```python
from build123d import *

# Parameters (mm, degrees)
F0_W          = 30
F0_H          = 42
F1_DEPTH      = 5
F2_T1_DEPTH   = 186.6590212458
F3_W          = 30
F3_H          = 2
F4_DEPTH      = 10
F5_W          = 35
F5_H          = 30
F6_DEPTH      = 5
F7_W          = 7
F7_H          = 30
F8_DEPTH      = 15
F9_R          = 2
F10_DEPTH     = 10
F11_R         = 4
F12_W         = 15
F12_H         = 14
F13_DEPTH     = 5
F14_W         = 15
F14_H         = 15
F15_DEPTH     = 5
F16_T4_DEPTH  = 35.8601958556
F16_T9_DEPTH  = 35.8601958556
F17_R         = 5
F18_T1_DEPTH  = 20
F18_T6_DEPTH  = 9.5699020722
F18_T11_DEPTH = 31.2132034356
F18_T16_DEPTH = 31.2132034356
F18_T21_DEPTH = 14
F18_T24_ANGLE = 90
F18_T26_ANGLE = 90
F18_T30_DEPTH = 13
F18_T36_DEPTH = 14
F18_T40_DEPTH = 31.2132034356
F18_T47_DEPTH = 13
F18_T51_DEPTH = 31.2132034356


# Not quite as in the source:
# - a fillet or chamfer that OpenCascade refuses, or shapes differently, is made with other operations: its cross-section is extruded or revolved along the edge and cut away or added


with BuildPart() as f1:
    # F0 (on Top) → F1 (new body)
    with BuildSketch(Plane.XY):
        with Locations((15, 21)):
            Rectangle(F0_W, F0_H)
    extrude(amount=F1_DEPTH)

    # F2: fillet of radius 37 on 1 edges, made by hand

    # F2_s2 → F2_t1 (cut)
    with BuildSketch(Plane.XY.offset(-90.8295106229)):
        with BuildLine():
            ThreePointArc((30, 5.6681957508), (21.5306852354, 29.2266337296), (0, 42))
            Line((0, 42), (30, 42))
            Line((30, 42), (30, 5.6681957508))
        make_face()
    extrude(amount=F2_T1_DEPTH, mode=Mode.SUBTRACT)

    # F3 (on face) → F4 (join)
    with BuildSketch(Plane.XY.offset(5)):
        with Locations((15, 1)):
            Rectangle(F3_W, F3_H)
    extrude(amount=F4_DEPTH)

    # F5 (on face) → F6 (join)
    with BuildSketch(Plane(origin=(0, 0, 0), x_dir=(0, -1, 0), z_dir=(-1, 0, 0))):
        with Locations((-25.5, 15)):
            Rectangle(F5_W, F5_H)
    extrude(amount=F6_DEPTH)

    # F7 (on face) → F8 (join)
    with BuildSketch(Plane(origin=(-5, 0, 0), x_dir=(0, -1, 0), z_dir=(-1, 0, 0))):
        with Locations((-11.5, 15)):
            Rectangle(F7_W, F7_H)
    extrude(amount=F8_DEPTH)

    # F9 (on face) → F10 (cut)
    with BuildSketch(Plane(origin=(0, 15, 0), x_dir=(-1, 0, 0), z_dir=(0, 1, 0))):
        with Locations((10, 15)):
            Circle(F9_R)
    extrude(amount=-F10_DEPTH, mode=Mode.SUBTRACT)

    # F11
    f11_edges = [f1.edges().sort_by_distance(p)[0] for p in [
        (21.530685, 29.226634, 0),
        (15, 0, 0),
    ]]
    fillet(f11_edges, radius=F11_R)

    # F12 (on face) → F13 (join)
    with BuildSketch(Plane(origin=(0, 0, 0), x_dir=(1, 0, 0), z_dir=(0, 0, -1))):
        with Locations((-12.5, -22)):
            Rectangle(F12_W, F12_H)
    extrude(amount=-F13_DEPTH)

    # F14 (on face) → F15 (join)
    with BuildSketch(Plane.XY.offset(30)):
        with Locations((-12.5, 22.5)):
            Rectangle(F14_W, F14_H)
    extrude(amount=-F15_DEPTH)

    # F16: chamfer of 15 on 2 edges, made by hand


with BuildPart() as f16_tool2:
    # F16_s3 → F16_t4 (new body)
    with BuildSketch(Plane.XY.offset(45.4300979278)):
        with BuildLine():
            Line((-20.4242640687, 14.5757359313), (-4.5757359313, 30.4242640687))
            Line((-4.5757359313, 30.4242640687), (-4.5757359313, 30.7242640687))
            ThreePointArc((-4.5757359313, 30.7242640687), (-12.2878679656, 30.3), (-20, 30.3))
            Line((-20, 30.3), (-20.3, 30))
            ThreePointArc((-20.3, 30), (-20.3, 22.2878679656), (-20.7242640687, 14.5757359313))
            Line((-20.7242640687, 14.5757359313), (-20.4242640687, 14.5757359313))
        make_face()
    extrude(amount=-F16_T4_DEPTH)

    split(bisect_by=Plane.YZ.offset(-5), keep=Keep.BOTTOM)


with BuildPart() as f1_1:
    add(f1.part)

    # F16_t1: cut F16_tool2
    add(f16_tool2.part, mode=Mode.SUBTRACT)


with BuildPart() as f16_tool7:
    # F16_s8 → F16_t9 (new body)
    with BuildSketch(Plane.XY.offset(-15.4300979278)):
        with BuildLine():
            Line((-4.5757359313, 29.4242640687), (-20.4242640687, 13.5757359313))
            Line((-20.4242640687, 13.5757359313), (-20.7242640687, 13.5757359313))
            ThreePointArc((-20.7242640687, 13.5757359313), (-20.3, 21.2878679656), (-20.3, 29))
            Line((-20.3, 29), (-20, 29.3))
            ThreePointArc((-20, 29.3), (-12.2878679656, 29.3), (-4.5757359313, 29.7242640687))
            Line((-4.5757359313, 29.7242640687), (-4.5757359313, 29.4242640687))
        make_face()
    extrude(amount=F16_T9_DEPTH)

    split(bisect_by=Plane.YZ.offset(-5), keep=Keep.BOTTOM)


with BuildPart() as f1_2:
    add(f1_1.part)

    # F16_t6: cut F16_tool7
    add(f16_tool7.part, mode=Mode.SUBTRACT)

    # F17
    f17_edges = [f1_2.edges().sort_by_distance(p)[0] for p in [
        (-2.5, 43, 0),
        (-2.5, 43, 30),
    ]]
    fillet(f17_edges, radius=F17_R)

    # F18: fillet of radius 2 on 9 edges, made by hand

    # F18_s2 → F18_t1 (cut)
    with BuildSketch(Plane.XY.offset(5)):
        with BuildLine():
            ThreePointArc((-3, 43), (-4.4142135624, 42.4142135624), (-5, 41))
            Line((-5, 41), (-5, 43))
            Line((-5, 43), (-3, 43))
        make_face()
    extrude(amount=F18_T1_DEPTH, mode=Mode.SUBTRACT)


with BuildPart() as f18_tool4:
    # F18_s5 → F18_t6 (new body)
    with BuildSketch(Plane.XY.offset(25)):
        with BuildLine():
            ThreePointArc((-20, 13), (-19.4142135624, 14.4142135624), (-18, 15))
            Line((-18, 15), (-20, 15))
            Line((-20, 15), (-20, 13))
        make_face()
    extrude(amount=-F18_T6_DEPTH)

    split(bisect_by=Plane(origin=(-17, 17, 0), x_dir=(0, 0, 1), z_dir=(-0.7071067812, 0.7071067812, 0)), keep=Keep.TOP)


with BuildPart() as f1_3:
    add(f1_2.part)

    # F18_t3: cut F18_tool4
    add(f18_tool4.part, mode=Mode.SUBTRACT)


with BuildPart() as f18_tool9:
    # F18_s10 → F18_t11 (new body)
    with BuildSketch(Plane(origin=(-6.5355339059, -6.5355339059, 0), x_dir=(0, 0, 1), z_dir=(0.7071067812, 0.7071067812, 0))):
        with BuildLine():
            ThreePointArc((0, -22.0416305603), (0.5857864376, -23.4558441227), (2, -24.0416305603))
            Line((2, -24.0416305603), (0, -24.0416305603))
            Line((0, -24.0416305603), (0, -22.0416305603))
        make_face()
    extrude(amount=F18_T11_DEPTH)

    split(bisect_by=Plane.YZ.offset(-5), keep=Keep.BOTTOM)


with BuildPart() as f1_4:
    add(f1_3.part)

    # F18_t8: cut F18_tool9
    add(f18_tool9.part, mode=Mode.SUBTRACT)


with BuildPart() as f18_tool14:
    # F18_s15 → F18_t16 (new body)
    with BuildSketch(Plane(origin=(16.0355339059, 16.0355339059, 0), x_dir=(0, 0, 1), z_dir=(-0.7071067812, -0.7071067812, 0))):
        with BuildLine():
            ThreePointArc((30, 22.7487373415), (29.4142135624, 24.1629509039), (28, 24.7487373415))
            Line((28, 24.7487373415), (30, 24.7487373415))
            Line((30, 24.7487373415), (30, 22.7487373415))
        make_face()
    extrude(amount=F18_T16_DEPTH)

    split(bisect_by=Plane.YZ.offset(-5), keep=Keep.BOTTOM)


with BuildPart() as f1_5:
    add(f1_4.part)

    # F18_t13: cut F18_tool14
    add(f18_tool14.part, mode=Mode.SUBTRACT)


with BuildPart() as f18_tool19:
    # F18_s20 → F18_t21 (new body)
    with BuildSketch(Plane.XZ.offset(-24)):
        with BuildLine():
            ThreePointArc((-3, 0), (-4.4142135624, 0.5857864376), (-5, 2))
            Line((-5, 2), (-5, 0))
            Line((-5, 0), (-3, 0))
        make_face()
    extrude(amount=-F18_T21_DEPTH)

    split(bisect_by=Plane(origin=(-17, 17, 0), x_dir=(0, 0, 1), z_dir=(-0.7071067812, 0.7071067812, 0)), keep=Keep.TOP)


with BuildPart() as f1_6:
    add(f1_5.part)

    # F18_t18: cut F18_tool19
    add(f18_tool19.part, mode=Mode.SUBTRACT)

    # F18_s23 → F18_t24 (revolve, cut)
    with BuildSketch(Plane.XY.offset(5)):
        with BuildLine():
            ThreePointArc((-3, 43), (-4.4142135624, 42.4142135624), (-5, 41))
            Line((-5, 41), (-5, 43))
            Line((-5, 43), (-3, 43))
        make_face()
    revolve(axis=Axis((-5, 38, 5), (-1, 0, 0)), revolution_arc=F18_T24_ANGLE, mode=Mode.SUBTRACT)

    # F18_s25 → F18_t26 (revolve, cut)
    with BuildSketch(Plane.XY.offset(25)):
        with BuildLine():
            ThreePointArc((-3, 43), (-4.4142135624, 42.4142135624), (-5, 41))
            Line((-5, 41), (-5, 43))
            Line((-5, 43), (-3, 43))
        make_face()
    revolve(axis=Axis((-5, 38, 25), (1, 0, 0)), revolution_arc=F18_T26_ANGLE, mode=Mode.SUBTRACT)


with BuildPart() as f18_tool28:
    # F18_s29 → F18_t30 (new body)
    with BuildSketch(Plane.XZ.offset(-25)):
        with BuildLine():
            ThreePointArc((-3, 30), (-4.4142135624, 29.4142135624), (-5, 28))
            Line((-5, 28), (-5, 30))
            Line((-5, 30), (-3, 30))
        make_face()
    extrude(amount=-F18_T30_DEPTH)

    split(bisect_by=Plane(origin=(-17.5, 17.5, 0), x_dir=(0, 0, 1), z_dir=(-0.7071067812, 0.7071067812, 0)), keep=Keep.TOP)


with BuildPart() as f1_7:
    add(f1_6.part)

    # F18_t27: cut F18_tool28
    add(f18_tool28.part, mode=Mode.SUBTRACT)


with BuildPart() as f18_tool34:
    # F18_s35 → F18_t36 (new body)
    with BuildSketch(Plane.XZ.offset(-24)):
        with BuildLine():
            ThreePointArc((-3, 0), (-4.4142135624, 0.5857864376), (-5, 2))
            Line((-5, 2), (-5, 0))
            Line((-5, 0), (-3, 0))
        make_face()
    extrude(amount=-F18_T36_DEPTH)

    split(bisect_by=Plane(origin=(-17, 17, 0), x_dir=(0, 0, 1), z_dir=(0.7071067812, -0.7071067812, 0)), keep=Keep.TOP)


with BuildPart() as f18_tool38:
    # F18_s39 → F18_t40 (new body)
    with BuildSketch(Plane(origin=(-6.5355339059, -6.5355339059, 0), x_dir=(0, 0, 1), z_dir=(0.7071067812, 0.7071067812, 0))):
        with BuildLine():
            ThreePointArc((0, -22.0416305603), (0.5857864376, -23.4558441227), (2, -24.0416305603))
            Line((2, -24.0416305603), (0, -24.0416305603))
            Line((0, -24.0416305603), (0, -22.0416305603))
        make_face()
    extrude(amount=F18_T40_DEPTH)

    split(bisect_by=Plane.YZ.offset(-5), keep=Keep.TOP)


with BuildPart() as f18_tool34_1:
    add(f18_tool34.part)

    # F18_t42: intersect F18_tool38
    add(f18_tool38.part, mode=Mode.INTERSECT)


with BuildPart() as f1_8:
    add(f1_7.part)

    # F18_t32: cut F18_tool34
    add(f18_tool34_1.part, mode=Mode.SUBTRACT)


with BuildPart() as f18_tool45:
    # F18_s46 → F18_t47 (new body)
    with BuildSketch(Plane.XZ.offset(-25)):
        with BuildLine():
            ThreePointArc((-3, 30), (-4.4142135624, 29.4142135624), (-5, 28))
            Line((-5, 28), (-5, 30))
            Line((-5, 30), (-3, 30))
        make_face()
    extrude(amount=-F18_T47_DEPTH)

    split(bisect_by=Plane(origin=(-17.5, 17.5, 0), x_dir=(0, 0, 1), z_dir=(0.7071067812, -0.7071067812, 0)), keep=Keep.TOP)


with BuildPart() as f18_tool49:
    # F18_s50 → F18_t51 (new body)
    with BuildSketch(Plane(origin=(16.0355339059, 16.0355339059, 0), x_dir=(0, 0, 1), z_dir=(-0.7071067812, -0.7071067812, 0))):
        with BuildLine():
            ThreePointArc((30, 22.7487373415), (29.4142135624, 24.1629509039), (28, 24.7487373415))
            Line((28, 24.7487373415), (30, 24.7487373415))
            Line((30, 24.7487373415), (30, 22.7487373415))
        make_face()
    extrude(amount=F18_T51_DEPTH)

    split(bisect_by=Plane.YZ.offset(-5), keep=Keep.TOP)


with BuildPart() as f18_tool45_1:
    add(f18_tool45.part)

    # F18_t53: intersect F18_tool49
    add(f18_tool49.part, mode=Mode.INTERSECT)


with BuildPart() as f1_9:
    add(f1_8.part)

    # F18_t43: cut F18_tool45
    add(f18_tool45_1.part, mode=Mode.SUBTRACT)


solid = f1_9.part
```
For this review, take the finished solid that the model builds, in its own axes (mm). A direction names the side the tool comes from. Round coordinates to 2 decimals unless told otherwise and drop trailing zeros. Write each loop counter-clockwise with the first axis right and the second up, starting at its lowest first coordinate (ties: lowest second). Pieces come first, ordered by that corner, then holes. Notation, with made-up numbers: (55, -25.5) - (103, -25.5) arc R22 ccw to (103, 8.5) - close; hole circle Ø7 at (-3, 38). An arc over 180 degrees is marked (long way). Answer as a JSON object with one key per item and string values.
1. We need section A-A on z = 6. Give the boundary of the cut face in (x, y), then the cut area to 3 significant figures.
Response values:
{"outline": "(-20, 8) - (0, 8) - (0, 43) - (-3, 43) arc R2 ccw to (-5, 41) - (-5, 15) - (-19, 15) - (-20, 14) - close; (0, 0) - (30, 0) - (30, 2) - (0, 2) - close", "area": "339 mm2"}
2. For pin 1 Ø6.5 at (x, z) = (-10, 15) entering from +Y; pin 2 Ø4 at (y, z) = (28.5, 13.5) entering from -X; pin 3 Ø11 at (x, z) = (22.5, 11) entering from +Y, all flat-tipped, find the tip position at first contact; note any pin that passes through.
Response values:
{"pin 1": "stops at y = 15", "pin 2": "stops at x = -5", "pin 3": "stops at y = 2"}
3. Tool access review of faces 4 (the face through (11, 18, 5)), 5 (the face through (0, 3, 4)), 6 (the face through (15, 2, 10)), 7 (the face through (-13, 15, 15)): name each direction out of +Z, -Z, +X, -X, +Y, -Y from which nothing blocks a thin tool from reaching the whole face with its end or side.
Response values:
{"face 4": "+Z, +X, +Y", "face 5": "+Z, -Z, -X, -Y", "face 6": "+Z, +X, -X, +Y", "face 7": "-X, +Y"}
4. Draft analysis for pull direction X (two halves, no side actions). For faces 1 (the face through (-10, 12, 17)), 2 (the face through (29.25, 3.42, 1.67)), 3 (the face through (-2, 41, 29)), state which applies: +X half, -X half, draft (parallel to the pull), parting line (faces both ways), or undercut.
Response values:
{"face 1": "undercut", "face 2": "+X half", "face 3": "draft"}
5. To check wall thickness, follow line 1 along Z through (x, y) = (-10, 12); line 2 along Z through (x, y) = (8, 31); line 3 along Y through (x, z) = (-8, 9.5). State the ranges of each line that lie inside material, in increasing order.
Response values:
{"line 1": "z = 0 to 13, 17 to 30", "line 2": "z = 0 to 5", "line 3": "y = 8 to 15"}
